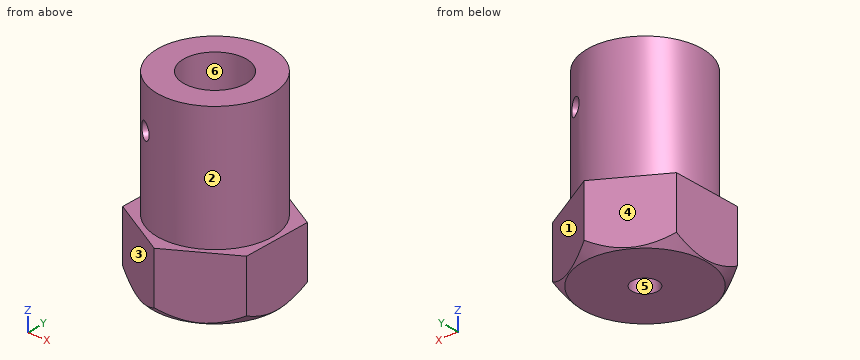
from build123d import *

# Parameters (mm, degrees)
EXTRUDE_1_DEPTH        = 6
SKETCH_2_R             = 5.5
EXTRUDE_2_DEPTH        = 12
HOLE_WIZARD_M3_1_D     = 2.5
HOLE_WIZARD_M3_1_DEPTH = 5.55
HOLE_WIZARD_M3_1_TIP   = 0.751075774
HOLE_WIZARD_M2_2_D     = 1.6
SKETCH_11_R            = 3
CUT_EXTRUDE_1_DEPTH    = 10


with BuildPart() as part:
    # 草图1 → 凸台-拉伸1 (new body)
    with BuildSketch(Plane.XY):
        Polygon((-6, 3.464101615), (0, 6.92820323), (6, 3.464101615), (6, -3.464101615), (0, -6.92820323), (-6, -3.464101615), align=None)
    extrude(amount=EXTRUDE_1_DEPTH)

    # 草图2 → 凸台-拉伸2 (add)
    with BuildSketch(Plane.XY.offset(6)):
        with Locations(Location((0, 0, 0), (0, 0, 180))):
            Circle(SKETCH_2_R)
    extrude(amount=EXTRUDE_2_DEPTH)

    # M3 螺纹孔1
    with Locations(Plane(origin=(0, 0, 0), x_dir=(-1, 0, 0), z_dir=(0, 0, -1))):
        with Locations((0, 0)):
            Hole(HOLE_WIZARD_M3_1_D / 2, depth=HOLE_WIZARD_M3_1_DEPTH)
            with Locations((0, 0, -(HOLE_WIZARD_M3_1_DEPTH + HOLE_WIZARD_M3_1_TIP / 2))):  # 118° drill point
                Cone(0, HOLE_WIZARD_M3_1_D / 2, HOLE_WIZARD_M3_1_TIP, mode=Mode.SUBTRACT)

    # M2 螺纹孔2 (through all)
    with Locations(Plane(origin=(-2.75, -4.763139721, 0), x_dir=(-0.866025403784438, 0.5000000000000011, 0), z_dir=(-0.5000000000000011, -0.8660254037844382, 0))):
        with Locations((0, -14)):
            Hole(HOLE_WIZARD_M2_2_D / 2)

    # 草图10 → 切除-旋转3 (revolve, cut)
    with BuildSketch(Plane(origin=(0, 0, 0), x_dir=(-0.866025403784438, 0.5000000000000011, 0), z_dir=(-0.5000000000000011, -0.8660254037844382, 0)), mode=Mode.PRIVATE) as cut_revolve_3_sk:
        Polygon((6.92820323, 0), (5.92820323, 0), (6.92820323, -1), align=None)
    revolve(cut_revolve_3_sk.sketch.rotate(Axis((0, 0, 0), (0, 0, 1)), 240.000000079), axis=Axis((0, 0, 0), (0, 0, 1)), mode=Mode.SUBTRACT)

    # 草图11 → 切除-拉伸1 (cut)
    with BuildSketch(Plane.XY.offset(18)):
        Circle(SKETCH_11_R)
    extrude(amount=-CUT_EXTRUDE_1_DEPTH, mode=Mode.SUBTRACT)


solid = part.part
Could you check a few things on this model? Use its own coordinates, in mm. Face numbers are marked on the shaded views. A direction names the side the tool comes from. Round coordinates to 2 decimals unless told otherwise and drop trailing zeros. Loops run counter-clockwise (first coordinate to the right, second up) from the corner with the lowest first, then second, coordinate; pieces in that order, holes last. Notation, with made-up numbers: (21, -30.5) - (38, -30.5) arc R13 cw to (38, -21.5) - close; hole circle Ø2 at (-26, -32.75). An arc over 180 degrees is marked (long way). Write item = value, one per line.
1) I'm going to push flat-ended pins straight in: P1, Ø6.5, axis at x = 1.5, y = 1, coming from the +Z side; P2, Ø6, axis at x = -4.5, z = 5, coming from the -Y side; P3, Ø4, axis at y = -4, z = 12.5, coming from the -X side; P4, Ø5, axis at x = 3.5, z = 8.5, coming from the -Y side. Where does each tip first touch, or does it pass through?
Computed:
P1 = 18
P2 = -6.06
P3 = -5.12
P4 = -5.41
2) On a 3-axis mill with a long thin cutter (end or side, diameter ignored), from which of +Z, -Z, +X, -X, +Y, -Y can I reach the whole of each face in a straight line? I mean the marked faces 1 and 2. Say none if no direction works.
Computed:
face_1 = +Z, -Z, +X, +Y
face_2 = +Z
3) If we mould it in two halves opening along Y, with no side actions, what happens to the marked faces 3, 4, 5 and 6? For each: pulls with the +Y half, pulls with the -Y half, needs draft (parallel to the pull), parting line crosses it, or undercut.
Computed:
face_3 = pulls with the -Y half
face_4 = pulls with the +Y half
face_5 = undercut
face_6 = undercut
4) Imagine slicing it at B-B (z = 14.25). Please give me the cut outline in (x, y).
Computed:
outline = (-3.38, -4.34) - (-2.11, -2.13) arc R3 cw to (0.79, 2.89) - (2.07, 5.1) arc R5.5 ccw to start; (-2.07, -5.1) arc R5.5 ccw to (3.38, 4.34) - (2.11, 2.13) arc R3 cw to (-0.79, -2.89) - close
5) I need wall thicknesses on line 1 along Y through (x, z) = (0, 14); line 2 along X through (y, z) = (0, 3.25); line 3 along Z through (x, y) = (1.25, 0.75). Which ranges of each line are inside material? Lowest first, please. Write a range as from..to.
Computed:
line_1 = -5.5..-3, 3..5.5
line_2 = -6..-1.25, 1.25..6
line_3 = 0..8
6) Imagine slicing it at A-A (z = 3.75). Please give me the cut outline in (x, y).
Computed:
outline = (-6, -3.46) - (0, -6.93) - (6, -3.46) - (6, 3.46) - (0, 6.93) - (-6, 3.46) - close; hole circle Ø2.5 at (0, 0)
7) Imagine slicing it at C-C (z = 10.25). Please give me the cut outline in (x, y), and give its area (3 significant figures).
Computed:
outline = circle Ø11 at (0, 0); hole circle Ø6 at (0, 0)
area = 66.8 mm2
